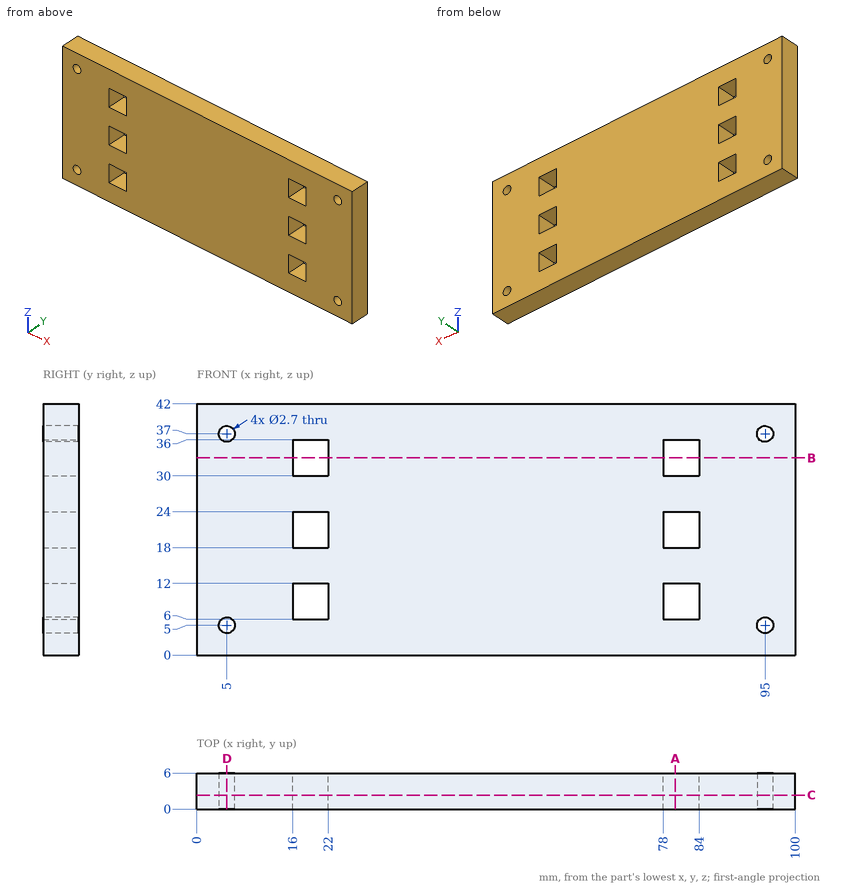
Input: dimensioned drawing with shaded views. Units: mm. Origin: part minimum x, y, z. Coordinates: 2 decimals unless noted, no trailing zeros. Loops run counter-clockwise (first coordinate to the right, second up) from the corner with the lowest first, then second, coordinate; pieces in that order, holes last. Notation, with made-up numbers: (50, 62) -> (93, 62) arc R25 ccw to (93, 88) -> close; hole circle Ø5 at (-20.75, 21.5). An arc over 180 degrees is marked (long way). One line per item, written item: value. Start each with the question number.
Q1. Line query: line 1 along X through (y, z) = (1.15, 23); line 2 along Z through (x, y) = (5, 4.1); line 3 along X through (y, z) = (2.75, 5). Output: solid intervals per line, ascending.
Q2. Section query B-B, the plane z = 33. Return the cut outline in (x, y), and give its area (3 significant figures).
Q3. Section query A-A, the plane x = 80. Return the cut outline in (y, z), and give its area (3 significant figures).
Q4. Section query C-C, the plane y = 2.35. Give the number of separate pieces and of enclosed holes in the cut face, and give its area (3 significant figures).
Q5. Section query D-D, the plane x = 5. Return the cut outline in (y, z).
Results:
1. line 1: 0 to 16, 22 to 78, 84 to 100
1. line 2: 0 to 3.65, 6.35 to 35.65, 38.35 to 42
1. line 3: 0 to 3.65, 6.35 to 93.65, 96.35 to 100
2. outline: (0, 0) -> (16, 0) -> (16, 6) -> (0, 6) -> close; (22, 0) -> (78, 0) -> (78, 6) -> (22, 6) -> close; (84, 0) -> (100, 0) -> (100, 6) -> (84, 6) -> close
2. area: 528 mm^2
3. outline: (0, 0) -> (6, 0) -> (6, 6) -> (0, 6) -> close; (0, 12) -> (6, 12) -> (6, 18) -> (0, 18) -> close; (0, 24) -> (6, 24) -> (6, 30) -> (0, 30) -> close; (0, 36) -> (6, 36) -> (6, 42) -> (0, 42) -> close
3. area: 144 mm^2
4. separate pieces: 1
4. enclosed holes: 10
4. area: 3,960 mm^2
5. outline: (0, 0) -> (6, 0) -> (6, 3.65) -> (0, 3.65) -> close; (0, 6.35) -> (6, 6.35) -> (6, 35.65) -> (0, 35.65) -> close; (0, 38.35) -> (6, 38.35) -> (6, 42) -> (0, 42) -> close
